Read the model definition and answer for the solid it produces. Units are mm, in the model's axes. Face numbers are marked on the shaded views. A direction names the side the tool comes from. Round coordinates to 2 decimals unless told otherwise and drop trailing zeros. Order: outer loops, then holes, each group sorted by start corner. A loop starts at its lowest first (then second) coordinate and runs counter-clockwise, first axis right, second up. Notation, with made-up numbers: (42.25, 12.5) -> (50.25, 12.5) arc R32 cw to (50.25, 47.5) -> close; hole circle Ø6 at (87, 47). An arc over 180 degrees is marked (long way). Use a Markdown table: item, result. Add a question column.
1. The mould has two halves that part along X. Classify the marked faces 1, 2 and 3: +X half, -X half, draft (parallel to the pull), parting line (faces both ways), or undercut.
2. Section B-B, the plane x = -5 is taken. Give the vertices of the cut face in (y, z), then the cut area to 3 significant figures.
3. For the marked faces 4 and 5, determine the directions among +Z, -Z, +X, -X, +Y, -Y from which every point of the face is accessible in a straight line to the end or side of a thin tool.
4. Section A-A, the plane y = 4 is taken. Give the vertices of the cut face in (x, z), then the cut area to 3 significant figures.
5. Consider L1, parallel to Y at x = -6, z = 12.5; L2, parallel to X at y = -10.5, z = 6. Determine where each line is inside the solid, lowest interval first. Write a range as [from, to].
6. Section C-C, the plane z = 2.5 is taken. Give the vertices of the cut face in (x, y), then the cut area to 3 significant figures.
```python
from build123d import *

# Parameters (mm, degrees)
SKETCH1_W           = 41
SKETCH1_H           = 47
SKETCH1_W_2         = 39
SKETCH1_H_2         = 45
BOSS_EXTRUDE1_DEPTH = 15
FILLET1_R           = 2
FILLET4_R           = 0.2


with BuildPart() as part:
    # Sketch1 → Boss-Extrude1 (new body)
    with BuildSketch(Plane.XY):
        Rectangle(SKETCH1_W, SKETCH1_H)
        Rectangle(SKETCH1_W_2, SKETCH1_H_2, mode=Mode.SUBTRACT)
    extrude(amount=BOSS_EXTRUDE1_DEPTH)

    # Fillet1
    fillet1_edges = [part.edges().sort_by_distance(p)[0] for p in [
        (-20.5, -23.5, 7.5),
        (-20.5, 23.5, 7.5),
        (20.5, 23.5, 7.5),
        (20.5, -23.5, 7.5),
    ]]
    fillet(fillet1_edges, radius=FILLET1_R)

    # Fillet4
    fillet4_edges = [part.edges().sort_by_distance(p)[0] for p in [
        (-19.5, 0, 0),
        (-19.5, 0, 15),
        (0, -23.5, 0),
        (0, -23.5, 15),
        (-20.5, 0, 0),
        (0, 23.5, 0),
        (20.5, 0, 0),
        (-19.914213562, 22.914213562, 0),
        (19.914213562, 22.914213562, 0),
        (19.914213562, -22.914213562, 0),
        (-19.914213562, -22.914213562, 0),
        (-20.5, 0, 15),
        (20.5, 0, 15),
        (0, 23.5, 15),
        (-19.914213562, 22.914213562, 15),
        (19.914213562, 22.914213562, 15),
        (19.914213562, -22.914213562, 15),
        (-19.914213562, -22.914213562, 15),
    ]]
    fillet(fillet4_edges, radius=FILLET4_R)


solid = part.part
```
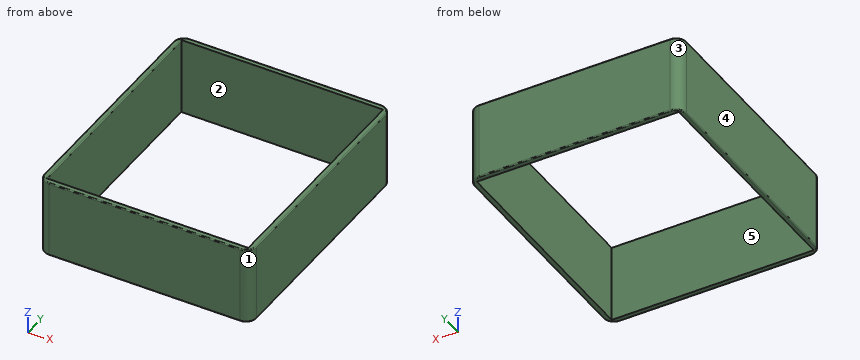
Verdict:
| question | item | result |
|---|---|---|
| 1 | face 1 | +X half |
| 1 | face 2 | undercut |
| 1 | face 3 | -X half |
| 2 | outline | (-23.5, 0.2) arc R0.2 ccw to (-23.3, 0) -> (-22.5, 0) -> (-22.5, 15) -> (-23.3, 15) arc R0.2 ccw to (-23.5, 14.8) -> close; (22.5, 0) -> (23.3, 0) arc R0.2 ccw to (23.5, 0.2) -> (23.5, 14.8) arc R0.2 ccw to (23.3, 15) -> (22.5, 15) -> close |
| 2 | area | 30.0 mm2 |
| 3 | face 4 | +Z, -Z, -X, +Y, -Y |
| 3 | face 5 | +Z, -Z |
| 4 | outline | (-20.5, 0.2) arc R0.2 ccw to (-20.3, 0) -> (-19.7, 0) arc R0.2 ccw to (-19.5, 0.2) -> (-19.5, 14.8) arc R0.2 ccw to (-19.7, 15) -> (-20.3, 15) arc R0.2 ccw to (-20.5, 14.8) -> close; (19.5, 0) -> (20.3, 0) arc R0.2 ccw to (20.5, 0.2) -> (20.5, 14.8) arc R0.2 ccw to (20.3, 15) -> (19.5, 15) -> close |
| 4 | area | 29.9 mm2 |
| 5 | L1 | y = [-23.5, -22.5], [22.5, 23.5] |
| 5 | L2 | x = [-20.5, -19.5], [19.5, 20.5] |
| 6 | outline | (-20.5, -21.5) arc R2 ccw to (-18.5, -23.5) -> (18.5, -23.5) arc R2 ccw to (20.5, -21.5) -> (20.5, 21.5) arc R2 ccw to (18.5, 23.5) -> (-18.5, 23.5) arc R2 ccw to (-20.5, 21.5) -> close; hole (-19.5, -22.5) -> (19.5, -22.5) -> (19.5, 22.5) -> (-19.5, 22.5) -> close |
| 6 | area | 169 mm2 |
